Check sheet for the modelled part. Datum: model origin and axes. Units: mm. A direction names the side the tool comes from. Give positions to 0.01 mm unless a question says otherwise; leave off trailing zeros. Order: outer loops, then holes, each group sorted by start corner. A loop starts at its lowest first (then second) coordinate and runs counter-clockwise, first axis right, second up.
```python
from build123d import *

# Parameters (mm, degrees)
F1_DEPTH  = 16
F2_R      = 7.99999
F3_R      = 1.55
F4_DEPTH  = 12.5
F5_DEPTH  = 25
F6_R      = 2.8
F7_DEPTH  = 3
F9_DEPTH  = 3
F10_R     = 1.125
F12_R     = 1.125
F15_DEPTH = 12.5
F17_DEPTH = 1.1


# Not quite as in the source:
# - a fillet or chamfer is up to 0.001 mm smaller than in the source, because OpenCascade refuses the exact size


with BuildPart() as f1:
    # F0 (on Front) → F1 (new body)
    with BuildSketch(Plane.XZ):
        Polygon((8, -18), (8, 18), (8, 26.5), (3.5, 26.5), (3.5, 13.9081878588), (-3.5, 13.9081878588), (-3.5, 26.5), (-8, 26.5), (-8, 18), (-8, -18), (-8, -26.5), (-3.5, -26.5), (-3.5, -18), (-3.5, -13), (3.5, -13), (3.5, -18), (3.5, -26.5), (8, -26.5), align=None)
    extrude(amount=F1_DEPTH)

    # F2 (radius 8 in the source; OpenCascade refuses exactly that, so slightly less here)
    f2_edges = [f1.edges().sort_by_distance(p)[0] for p in [
        (5.75, -16, 26.5),
        (-5.75, -16, 26.5),
        (-5.75, 0, 26.5),
        (5.75, 0, 26.5),
        (5.75, -16, -26.5),
        (-5.75, -16, -26.5),
        (5.75, 0, -26.5),
        (-5.75, 0, -26.5),
    ]]
    fillet(f2_edges, radius=F2_R)

    # F3 (on face) → F4 (cut, symmetric)
    with BuildSketch(Plane.YZ.offset(8)):
        with Locations((-8, 19.8896080256)):
            Circle(F3_R)
        with Locations((-8, -19.8896080256)):
            Circle(F3_R)
    extrude(amount=F4_DEPTH, both=True, mode=Mode.SUBTRACT)

    # F3 (on face) → F5 (cut)
    with BuildSketch(Plane.YZ.offset(8)):
        with Locations((-8, 19.8896080256)):
            Circle(F3_R)
        with Locations((-8, -19.8896080256)):
            Circle(F3_R)
    extrude(amount=-F5_DEPTH, mode=Mode.SUBTRACT)

    # F6 (on face) → F7 (cut)
    with BuildSketch(Plane.YZ.offset(8)):
        with Locations((-8, 19.8896080256)):
            Circle(F6_R)
        with Locations((-8, -19.8896080256)):
            Circle(F6_R)
    extrude(amount=-F7_DEPTH, mode=Mode.SUBTRACT)

    # F8 (on face) → F9 (cut)
    with BuildSketch(Plane(origin=(-8, 0, 0), x_dir=(0, -1, 0), z_dir=(-1, 0, 0))):
        Polygon((10.75, 18.3018947853), (10.75, 21.4773212658), (8, 23.0650345061), (5.25, 21.4773212658), (5.25, 18.3018947853), (8, 16.714181545), align=None)
        Polygon((5.25, -18.3018947853), (5.25, -21.4773212658), (8, -23.0650345061), (10.75, -21.4773212658), (10.75, -18.3018947853), (8, -16.714181545), align=None)
    extrude(amount=-F9_DEPTH, mode=Mode.SUBTRACT)

    # F10 (on face) → F11 (revolve)
    with BuildSketch(Plane.XZ.offset(16)):
        with Locations((-3, 0)):
            Circle(F10_R)
    revolve(axis=Axis((0, -16, 0.0619328348), (0, 0, -1)))

    # F12 (on face) → F13 (revolve)
    with BuildSketch(Plane(origin=(0, 0, 0), x_dir=(-1, 0, 0), z_dir=(0, 1, 0))):
        with Locations((3, 0)):
            Circle(F12_R)
    revolve(axis=Axis((0, 0, 0.5132202059), (0, 0, -1)))

    # F14 (on Top) → F15 (cut, symmetric)
    with BuildSketch(Plane.XY):
        Polygon((1.875, -16), (-1.875, -16), (-4.125, -16), (-8, -16), (-8, -21.5492993593), (8, -21.5492993593), (8, -16), (4.125, -16), align=None)
    extrude(amount=F15_DEPTH, both=True, mode=Mode.SUBTRACT)

    # F16 (on Right) → F17 (cut, symmetric)
    with BuildSketch(Plane.YZ):
        with BuildLine():
            Line((-16, -5.4295487842), (-16, -8.2849260709))
            ThreePointArc((-16, -8.2849260709), (-11.6, 0), (-16, 8.2849260709))
            Line((-16, 8.2849260709), (-16, 5.4295487842))
            ThreePointArc((-16, 5.4295487842), (-13.8, 0), (-16, -5.4295487842))
        make_face()
    extrude(amount=F17_DEPTH, both=True, mode=Mode.SUBTRACT)


solid = f1.part
```
(1) Gauge pin test, flat ends, axial feed: pin 1 Ø6 at (x, z) = (-3, -19.5) entering from +Y; pin 2 Ø1 at (x, y) = (-1.5, -8) entering from +Z; pin 3 Ø2.5 at (x, z) = (-6, 20) entering from -Y. Record the tip position at first contact, or that the pin passes through.
Response values:
pin 1: stops at y = 0
pin 2: stops at z = 13.91
pin 3: stops at y = -16
(2) Cross-section at C-C on y = -12.75. Enter the section's corners in (x, z), then the cut area to 3 significant figures.
Response values:
outline: (-8, -24.94) - (-3.5, -24.94) - (-3.5, -13) - (3.5, -13) - (3.5, -24.94) - (8, -24.94) - (8, 24.94) - (3.5, 24.94) - (3.5, 13.91) - (-3.5, 13.91) - (-3.5, 24.94) - (-8, 24.94) - close; hole (-1.1, -4.66) - (1.1, -4.66) - (1.1, 4.66) - (-1.1, 4.66) - close
area: 617 mm2
(3) Cross-section at D-D on z = -4. Enter the section's corners in (x, y), then the cut area to 3 significant figures.
Response values:
outline: (-8, -16) - (8, -16) - (8, 0) - (-8, 0) - close; hole (-1.1, -14.9) - (1.1, -14.9) - (1.1, -12.43) - (-1.1, -12.43) - close
area: 251 mm2
(4) Cross-section at B-B on x = -6.75. Count the separate pieces of the cut face and the enclosed holes in it, then the cut area to 3 significant figures.
Response values:
separate pieces: 1
enclosed holes: 2
area: 741 mm2
(5) Set-up check for faces 4 (the face through (0, -8, -13)), 5 (the face through (-6.521, -9.394, 22.26)), 6 (the face through (6.521, -5.414, 18.817)), 7 (the face through (0, -11.6, -0.1)): record each of +Z, -Z, +X, -X, +Y, -Y from which the full face is reachable in a straight line by a thin tool's end or side.
Response values:
face 4: -Z, +Y, -Y
face 5: -X
face 6: +X
face 7: none
(6) Release check for a two-part mould opening along Y. For faces 1 (the face through (-5, -9.2, 18.5)), 2 (the face through (5.719, -13.594, 24.219)), 3 (the face through (-8, -8, 0)) record: released by +Y, released by -Y, zero draft, split by the parting line, or undercut.
Response values:
face 1: undercut
face 2: released by -Y
face 3: zero draft
(7) Cross-section at A-A on z = -16. Enter the section's corners in (x, y).
Response values:
outline: (-8, -16) - (-3.5, -16) - (-3.5, 0) - (-8, 0) - close; (3.5, -16) - (8, -16) - (8, 0) - (3.5, 0) - close
(8) Material ranges on L1, parallel to Z at x = 3.9, y = -8; L2, parallel to Z at x = -6.75, y = -8; L3, parallel to X at y = -6.25, z = 17, recorded low to high.
Response values:
L1: z = -26.5 to -21.44, -18.34 to 18.34, 21.44 to 26.5
L2: z = -26.5 to -23.07, -16.71 to 16.71, 23.07 to 26.5
L3: x = -8 to -3.5, 3.5 to 8
